Work out the finished part from the listing and answer in its coordinate system (mm). A direction names the side the tool comes from. Coordinates: 2 decimals unless noted, no trailing zeros. Write each loop counter-clockwise with the first axis right and the second up, starting at its lowest first coordinate (ties: lowest second). Pieces come first, ordered by that corner, then holes. Notation, with made-up numbers: (24.5, 6) - (48.5, 6) arc R31 ccw to (48.5, 40) - close; hole circle Ø2 at (55.25, 20.25). An arc over 180 degrees is marked (long way). Use CSV: the item, a comma, the result in double quotes. Start each with the question number.
from build123d import *

# Parameters (mm, degrees)
F0_R     = 10
F1_DEPTH = 14
F2_R     = 3
F3_DEPTH = 12
F4_R     = 10
F4_R_2   = 9.5
F5_DEPTH = 1.5


with BuildPart() as f1:
    # F0 (on Top) → F1 (new body)
    with BuildSketch(Plane.XY):
        Circle(F0_R)
    extrude(amount=F1_DEPTH)

    # F2 (on face) → F3 (cut)
    with BuildSketch(Plane(origin=(0, 0, 0), x_dir=(1, 0, 0), z_dir=(0, 0, -1))):
        Circle(F2_R)
    extrude(amount=-F3_DEPTH, mode=Mode.SUBTRACT)

    # F4 (on face) → F5 (cut)
    with BuildSketch(Plane.XY.offset(14)):
        Circle(F4_R)
        Circle(F4_R_2, mode=Mode.SUBTRACT)
    extrude(amount=-F5_DEPTH, mode=Mode.SUBTRACT)


solid = f1.part
Item 1: Straight lines are drawn through the part: probe 1 along Y at (x, z) = (0, 7.5); probe 2 along Z at (x, y) = (1.5, -1); probe 3 along Y at (x, z) = (-1.5, 7). For each, find the intervals that lie inside material, in ascending order. Write a range as [from, to].
Item 2: Each of these flat-tipped pins is pushed along its axis until it touches: pin 1 (10 mm diameter, centred on x = -4, y = -2, fed in from -Z); pin 2 (4 mm diameter, centred on x = 3, z = 4, fed in from +Y); pin 3 (6 mm diameter, centred on x = 7, z = 8, fed in from +Y). Where does it stop, or does it pass through?
Item 3: A cutting plane is placed at A-A (y = 0). Determine the outline of the cut face in (x, z).
Item 4: Which of the six approach directions +Z, -Z, +X, -X, +Y, -Y give full straight-line access (tool end or side, diameter ignored) to faces 5 (the face through (0, 0, 14)), 6 (the face through (4.38, -8.43, 13.26))?
Item 5: A cutting plane is placed at D-D (x = -8.25). Determine the outline of the cut face in (y, z), then the cut area to 3 significant figures.
Item 6: Determine the mould class of faces 1 (the face through (-3, 0, 6)), 2 (the face through (9, -4, 12.5)), 3 (the face through (-2.17, -9.76, 6.16)), 4 (the face through (0, 0, 12)) for opening direction X: +X half, -X half, draft (parallel to the pull), parting line (faces both ways), or undercut.
Item 7: A cutting plane is placed at C-C (z = 3.25). Determine the outline of the cut face in (x, y), then the cut area to 3 significant figures.
Calculated:
1,probe 1,"y = [-10, -3], [3, 10]"
1,probe 2,"z = [12, 14]"
1,probe 3,"y = [-9.89, -2.6], [2.6, 9.89]"
2,pin 1,"stops at z = 0"
2,pin 2,"stops at y = 9.95"
2,pin 3,"stops at y = 9.17"
3,outline,"(-10, 0) - (-3, 0) - (-3, 12) - (3, 12) - (3, 0) - (10, 0) - (10, 12.5) - (9.5, 12.5) - (9.5, 14) - (-9.5, 14) - (-9.5, 12.5) - (-10, 12.5) - close"
4,face 5,"+Z, +X, -X, +Y, -Y"
4,face 6,"+Z"
5,outline,"(-5.65, 0) - (5.65, 0) - (5.65, 12.5) - (4.71, 12.5) - (4.71, 14) - (-4.71, 14) - (-4.71, 12.5) - (-5.65, 12.5) - close"
5,area,"155 mm²"
6,face 1,"undercut"
6,face 2,"draft"
6,face 3,"parting line"
6,face 4,"undercut"
7,outline,"circle Ø20 at (0, 0); hole circle Ø6 at (0, 0)"
7,area,"286 mm²"
